from build123d import *

# Parameters (mm, degrees)
SKETCH1_W                = 40
SKETCH1_H                = 40
BOSS_EXTRUDE1_DEPTH      = 40
SKETCH2_W                = 25
SKETCH2_H                = 20
CUT_EXTRUDE1_DEPTH       = 40
CHAMFER1_SIZE            = 15
CUT_EXTRUDE2_DEPTH       = 15
CHAMFER2_SIZE            = 4
SKETCH4_R                = 2.6
CUT_EXTRUDE3_DEPTH       = 17
BOSS_EXTRUDE3_DEPTH      = 20
FILLET3_R                = 4
BOSS_EXTRUDE2_DEPTH      = 20
BOSS_EXTRUDE2_DEPTH_BACK = 25
SKETCH5_W                = 50
SKETCH5_H                = 8
SKETCH10_R               = 14
CUT_EXTRUDE4_DEPTH       = 10
CHAMFER3_SIZE            = 15
CHAMFER3_SIZE_2          = 20
CHAMFER4_SIZE2           = 50
CHAMFER4_SIZE            = 15
FILLET5_START            = 26
FILLET5_DEPTH            = 10
FILLET6_R                = 2
CHAMFER5_SIZE            = 22
SKETCH11_W               = 27.237482008
SKETCH11_H               = 25
CUT_EXTRUDE5_DEPTH       = 25
FILLET7_R                = 4
SKETCH16_W               = 14
SKETCH16_H               = 14
CUT_EXTRUDE6_DEPTH       = 43
CHAMFER6_SIZE            = 10
CHAMFER6_SIZE2           = 2
FILLET9_R                = 2
SKETCH18_W               = 50
SKETCH18_H               = 14
BOSS_EXTRUDE4_DEPTH      = 25
SKETCH19_R               = 2.25
CUT_EXTRUDE7_DEPTH       = 15
FILLET10_R               = 5
SKETCH20_W               = 50
SKETCH20_H               = 1
CUT_EXTRUDE8_DEPTH       = 69
FILLET11_R               = 10
SKETCH21_R               = 14
CUT_EXTRUDE9_DEPTH       = 69


with BuildPart() as part:
    # Sketch1 → Boss-Extrude1 (new body)
    with BuildSketch(Plane(origin=(0, 0, 0), x_dir=(1, 0, 0), z_dir=(0, 1, 0))):
        with Locations((20, 20)):
            Rectangle(SKETCH1_W, SKETCH1_H)
    extrude(amount=BOSS_EXTRUDE1_DEPTH)

    # Sketch2 → Cut-Extrude1 (cut)
    with BuildSketch(Plane(origin=(0, 40, 0), x_dir=(1, 0, 0), z_dir=(0, 1, 0))):
        with Locations((12.5, 30)):
            Rectangle(SKETCH2_W, SKETCH2_H)
    extrude(amount=-CUT_EXTRUDE1_DEPTH, mode=Mode.SUBTRACT)

    # Chamfer1
    chamfer1_edges = [part.edges().sort_by_distance(p)[0] for p in [
        (0, 20, 0),
    ]]
    chamfer(chamfer1_edges, length=CHAMFER1_SIZE)

    # Sketch3 → Cut-Extrude2 (cut)
    with BuildSketch(Plane.XY):
        Polygon((0, 10), (0, 15), (15, 15), (15, 5), (0, 5), align=None)
        Polygon((0, 30), (0, 25), (15, 25), (15, 35), (0, 35), align=None)
    extrude(amount=-CUT_EXTRUDE2_DEPTH, mode=Mode.SUBTRACT)

    # Chamfer2
    chamfer2_edges = [part.edges().sort_by_distance(p)[0] for p in [
        (15, 35, -7.5),
        (15, 25, -7.5),
        (15, 15, -7.5),
        (15, 5, -7.5),
    ]]
    chamfer(chamfer2_edges, length=CHAMFER2_SIZE)

    # Sketch4 → Cut-Extrude3 (cut)
    with BuildSketch(Plane.XY.offset(-15)):
        with Locations((8, 30)):
            Circle(SKETCH4_R)
        with Locations((8, 10)):
            Circle(SKETCH4_R)
    extrude(amount=-CUT_EXTRUDE3_DEPTH, mode=Mode.SUBTRACT)

    # Sketch9 → Boss-Extrude3 (add)
    with BuildSketch(Plane(origin=(40, 0, 0), x_dir=(0, 0, -1), z_dir=(1, 0, 0))):
        Polygon((0, 40), (0, 55), (4, 55), (20, 40), align=None)
        Polygon((0, 0), (0, -15), (4, -15), (20, 0), align=None)
    extrude(amount=-BOSS_EXTRUDE3_DEPTH)

    # Fillet3
    fillet3_edges = [part.edges().sort_by_distance(p)[0] for p in [
        (20, 55, -2),
        (40, 55, -2),
        (20, -15, -2),
        (40, -15, -2),
    ]]
    fillet(fillet3_edges, radius=FILLET3_R)

    # Sketch5 → Boss-Extrude2 (add, two sides: drawn at the far end of the back side and taken through both)
    with BuildSketch(Plane(origin=(0, 0, -40), x_dir=(-1, 0, 0), z_dir=(0, 0, -1)).offset(-BOSS_EXTRUDE2_DEPTH_BACK)):
        with Locations((-65, 31)):
            Rectangle(SKETCH5_W, SKETCH5_H)
    extrude(amount=BOSS_EXTRUDE2_DEPTH + BOSS_EXTRUDE2_DEPTH_BACK)

    # Sketch10 → Cut-Extrude4 (cut)
    with BuildSketch(Plane(origin=(0, 27, 0), x_dir=(-1, 0, 0), z_dir=(0, -1, 0))):
        with Locations(Location((-66.5, 38, 0), (0, 0, 90))):
            Circle(SKETCH10_R)
    extrude(amount=-CUT_EXTRUDE4_DEPTH, mode=Mode.SUBTRACT)

    # Chamfer3
    # the kernel refuses this chamfer: 20, 15 mm, written as the material it adds along each edge
    with BuildSketch(Plane(origin=(40, 27, -40), x_dir=(-1, 0, 0), z_dir=(0, 1, 0))) as chamfer3_piece_1:
        Polygon((CHAMFER3_SIZE, 0), (0, -CHAMFER3_SIZE_2), (0, 0), align=None)
    extrude(amount=8)

    # Chamfer4
    chamfer4_edges = [part.edges().sort_by_distance(p)[0] for p in [
        (40, 31, -15),
    ]]
    chamfer4_side = [part.faces().sort_by_distance(p)[0] for p in [
        (40, 31, -14.7),
    ]]
    chamfer(chamfer4_edges, length=CHAMFER4_SIZE - 0.0001, length2=CHAMFER4_SIZE2 - 0.0001, reference=chamfer4_side[0])  # a hair under: the kernel refuses the full size

    # Fillet5: read off the stored shape, not the designer's step
    # Fillet5 outline → Fillet5 (cut)
    with BuildSketch(Plane(origin=(0, 0, 0), x_dir=(1, 0, 0), z_dir=(0, 1, 0)).offset(FILLET5_START)):
        with BuildLine():
            Line((90, 15), (90, 17.976122604))
            ThreePointArc((90, 17.976122604), (89.209171713, 15.588400485), (87.149391542, 14.144817463))
            Line((87.149391542, 14.144817463), (90, 15))
        make_face()
        with BuildLine():
            ThreePointArc((38.8, 58.4), (40.211145618, 59.577708764), (42, 60))
            Line((42, 60), (40, 60))
            Line((40, 60), (38.8, 58.4))
        make_face()
        with BuildLine():
            ThreePointArc((86, 60), (88.828427125, 58.828427125), (90, 56))
            Line((90, 56), (90, 60))
            Line((90, 60), (86, 60))
        make_face()
    extrude(amount=FILLET5_DEPTH, mode=Mode.SUBTRACT)

    # Fillet6
    fillet6_edges = [part.edges().sort_by_distance(p)[0] for p in [
        (32.5, 40, -40),
        (32.5, 0, -40),
    ]]
    fillet(fillet6_edges, radius=FILLET6_R)

    # Chamfer5
    # the kernel refuses this chamfer: 22 mm, written as the material it adds along each edge
    with BuildSketch(Plane(origin=(40, 27, 56.576925735), x_dir=(1, 0, 0), z_dir=(0, 0, -1))) as chamfer5_piece_1_section:
        Polygon((CHAMFER5_SIZE, 0), (0, CHAMFER5_SIZE), (0, 0), align=None)
    chamfer5_piece_1 = extrude(amount=96.576925735, mode=Mode.PRIVATE)
    chamfer5_piece_1 = split(chamfer5_piece_1, bisect_by=Plane(origin=(24.428402209, 27, 4.671357537), z_dir=(-0.2873466553275782, 0, -0.9578266542919204)), keep=Keep.TOP, mode=Mode.PRIVATE)
    chamfer5_piece_1 = chamfer5_piece_1 - Plane(origin=(66.5, 27, -38), x_dir=(0, 0, -1), z_dir=(0, -1, 0)) * Cylinder(14, 282, mode=Mode.PRIVATE)
    chamfer5_piece_1 = split(chamfer5_piece_1, bisect_by=Plane(origin=(40, 27, 0), z_dir=(0, 0, -1)), keep=Keep.TOP, mode=Mode.PRIVATE)
    add(chamfer5_piece_1)

    # Sketch11 → Cut-Extrude5 (cut)
    with BuildSketch(Plane(origin=(0, 0, -40), x_dir=(-1, 0, 0), z_dir=(0, 0, -1))):
        with Locations((-53.618741004, 14.5)):
            Rectangle(SKETCH11_W, SKETCH11_H)
    extrude(amount=-CUT_EXTRUDE5_DEPTH, mode=Mode.SUBTRACT)

    # Fillet7
    fillet7_edges = [part.edges().sort_by_distance(p)[0] for p in [
        (62, 27, -10.8000346),
        (40, 5, -7.50005),
    ]]
    fillet(fillet7_edges, radius=FILLET7_R)

    # Sketch16 → Cut-Extrude6 (cut)
    with BuildSketch(Plane.ZY):
        with Locations((-29, 20)):
            Rectangle(SKETCH16_W, SKETCH16_H)
    extrude(amount=-CUT_EXTRUDE6_DEPTH, mode=Mode.SUBTRACT)

    # Chamfer6
    chamfer6_edges = [part.edges().sort_by_distance(p)[0] for p in [
        (40, 20, -36),
    ]]
    chamfer6_side = [part.faces().sort_by_distance(p)[0] for p in [
        (32.5, 20, -36),
    ]]
    chamfer(chamfer6_edges, length=CHAMFER6_SIZE, length2=CHAMFER6_SIZE2, reference=chamfer6_side[0])

    # Fillet9
    fillet9_edges = [part.edges().sort_by_distance(p)[0] for p in [
        (32.5, 13, -22),
        (32.5, 27, -22),
        (27.5, 27, -36),
        (27.5, 13, -36),
        (35, 13, -37),
        (35, 27, -37),
    ]]
    fillet(fillet9_edges, radius=FILLET9_R)

    # Sketch18 → Boss-Extrude4 (add)
    with BuildSketch(Plane.XY):
        with Locations((65, 42)):
            Rectangle(SKETCH18_W, SKETCH18_H)
    extrude(amount=-BOSS_EXTRUDE4_DEPTH)

    # Sketch19 → Cut-Extrude7 (cut)
    with BuildSketch(Plane(origin=(0, 0, -25), x_dir=(-1, 0, 0), z_dir=(0, 0, -1))):
        with Locations((-79.5, 45)):
            Circle(SKETCH19_R)
        with Locations(Location((-79.5, 37, 0), (0, 0, 297.266044451))):
            Circle(SKETCH19_R)
        with Locations((-53.5, 45)):
            Circle(SKETCH19_R)
        with Locations((-53.5, 37)):
            Circle(SKETCH19_R)
    extrude(amount=-CUT_EXTRUDE7_DEPTH, mode=Mode.SUBTRACT)

    # Fillet10
    fillet10_edges = [part.edges().sort_by_distance(p)[0] for p in [
        (90, 35, -8.988061302),
        (90, 49, -12.5),
        (40, 49, -17.7),
    ]]
    fillet(fillet10_edges, radius=FILLET10_R)

    # Sketch20 → Cut-Extrude8 (cut)
    with BuildSketch(Plane(origin=(0, 0, -25), x_dir=(-1, 0, 0), z_dir=(0, 0, -1))):
        with Locations((-65, 34.5)):
            Rectangle(SKETCH20_W, SKETCH20_H)
    extrude(amount=CUT_EXTRUDE8_DEPTH, mode=Mode.SUBTRACT)

    # Fillet11
    # the kernel refuses this fillet: 10 mm, written as the material it takes off along each edge
    with BuildSketch(Plane(origin=(40, 35, -40), x_dir=(-1, 0, 0), z_dir=(0, 0, -1))) as fillet11_piece_1:
        with BuildLine():
            CenterArc((4.358898944, -10), FILLET11_R, 90, 25.841932763)
            Line((0, -1), (0, 0))
            Line((0, 0), (4.358898944, 0))
        make_face()
    extrude(amount=30.361348974, mode=Mode.SUBTRACT)

    # Sketch21 → Cut-Extrude9 (cut)
    with BuildSketch(Plane.XZ.offset(-35)):
        with Locations(Location((66.5, -38, 0), (0, 0, 270))):
            Circle(SKETCH21_R)
    extrude(amount=-CUT_EXTRUDE9_DEPTH, mode=Mode.SUBTRACT)


solid = part.part
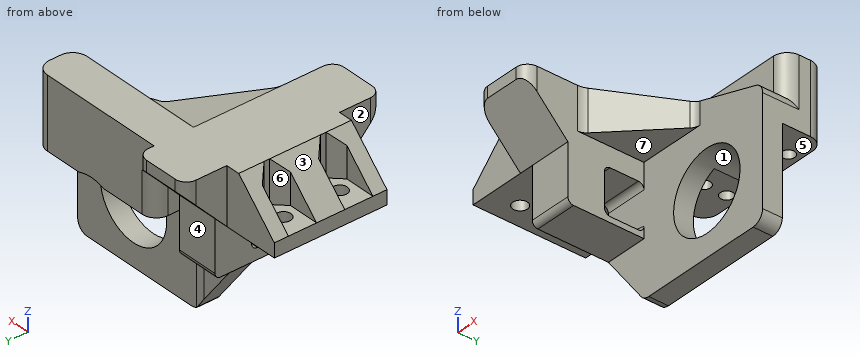
Can you work these out from the model? Positions are in its coordinate system, mm. Face numbers are marked on the shaded views. A direction names the side the tool comes from. Coordinates: 2 decimals unless noted, no trailing zeros. Loops run counter-clockwise (first coordinate to the right, second up) from the corner with the lowest first, then second, coordinate; pieces in that order, holes last. Notation, with made-up numbers: M -23.5,39.5 L 20.5,39.5 A18 cw 20.5,47.5 Z; hole C -31,21 d8. An arc over 180 degrees is marked long. Return JSON: item names as keys, results as strings. Group by question number.
Item 1: I'm going to push flat-ended pins straight in: pin 1 Ø12.5 at (x, y) = (18, 14) entering from -Z; pin 2 Ø3 at (x, z) = (28.5, -50) entering from +Y; pin 3 Ø10 at (x, z) = (8.5, -11) entering from -Y; pin 4 Ø5 at (y, z) = (37, -34.5) entering from +X. Where does each tip first touch, or does it pass through?
Item 2: Imagine slicing it at C-C (x = 50). Please give me the cut outline in (y, z), and give its area (3 significant figures).
Item 3: Imagine slicing it at D-D (x = 18.5). Please give me the cut outline in (y, z).
Item 4: Imagine slicing it at B-B (z = -50.5). Please give me the cut outline in (x, y) (3 decimals).
Item 5: Imagine slicing it at A-A (x = 9). Please give me the cut outline in (y, z).
Item 6: On a 3-axis mill with a long thin cutter (end or side, diameter ignored), from which of +Z, -Z, +X, -X, +Y, -Y can I reach the whole of each face in a straight line? I mean the marked faces 4, 5, 6 and 7. Say none if no direction works.
Item 7: If I drill on L1, parallel to X at y = 37, z = -20.5; L2, parallel to Y at x = 53.5, z = -19.5; L3, parallel to Y at x = 9, z = -19.5, over which ranges is the centre line in solid material (lowest first)? Write a range as from..to.
Item 8: Thinking about a two-plate mould opening in Z: for the marked faces 1, 2 and 3, which applies, released by +Z, released by -Z, zero draft, split by the parting line, or undercut?
Verdict:
{
 "1": {"pin 1": "stops at z = -20", "pin 2": "passes through", "pin 3": "stops at y = 0", "pin 4": "stops at x = 40"},
 "2": {"outline": "M 15,-15 L 27,-15 L 27,-60 L 34,-60 L 34,-25 L 49,-25 L 49,0 L 35,0 L 35,-3 L 15,-3 Z", "area": "915 mm^2"},
 "3": {"outline": "M 0,-20 L 40,-20 L 40,0 L 0,0 Z"},
 "4": {"outline": "M 32.875,27 L 60.195,27 L 60.195,34 L 40,34 A10 ccw 35.641,35 L 32.875,35 Z; M 72.805,27 L 90,27 L 90,34 L 72.805,34 Z"},
 "5": {"outline": "M 0,-20 L 7.6,-20 L 7.6,-15 L 5,-15 L 5,-6 L 0,-6 Z; M 12.4,-20 L 27.6,-20 L 27.6,-15 L 25,-15 L 25,-6 L 15,-6 L 15,-15 L 12.4,-15 Z; M 32.4,-20 L 40,-20 L 40,-6 L 35,-6 L 35,-15 L 32.4,-15 Z"},
 "6": {"face 4": "-Z, -X, +Y", "face 5": "-Z, +X, +Y", "face 6": "+Z, -X", "face 7": "-Z, +X, -Y"},
 "7": {"L1": "x = 25..51.25, 55.75..77.25, 81.75..90", "L2": "y = 27..34.75, 39.25..42.75, 47.25..49", "L3": "y = 0..7.6, 12.4..27.6, 32.4..40"},
 "8": {"face 1": "undercut", "face 2": "zero draft", "face 3": "released by +Z"}
}
